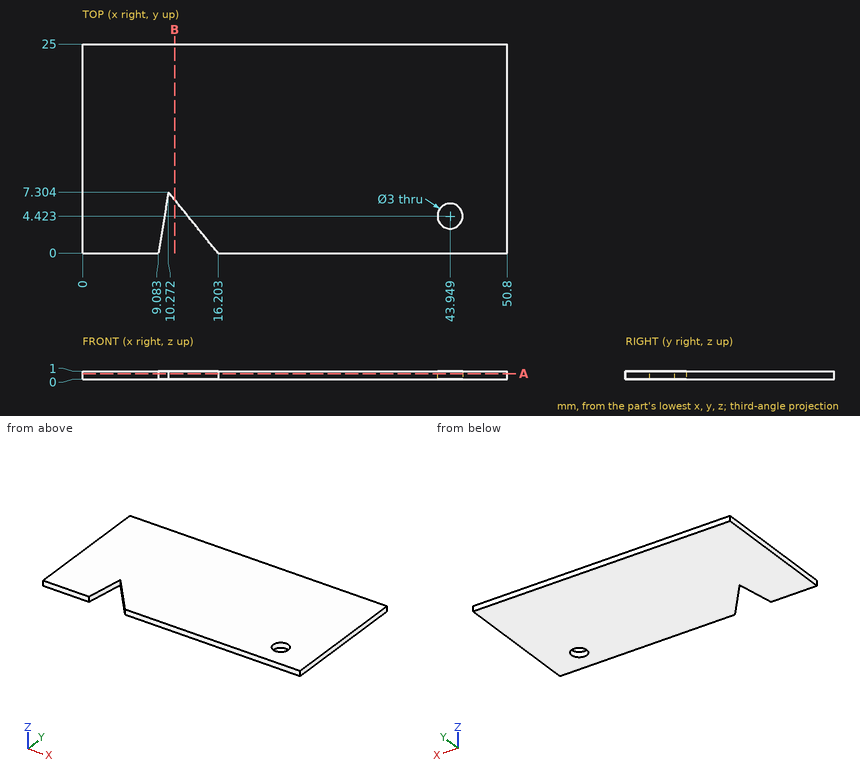
Input: dimensioned drawing with shaded views. Units: mm. Origin: part minimum x, y, z. Coordinates: 2 decimals unless noted, no trailing zeros. Order: outer loops, then holes, each group sorted by start corner. A loop starts at its lowest first (then second) coordinate and runs counter-clockwise, first axis right, second up.
Item 1: Section query B-B (x = 11). Output: boundary loops of the cut face in (y, z), then the cut area to 3 significant figures.
Answer:
outline: (6.41, 0) - (25, 0) - (25, 1) - (6.41, 1) - close
area: 18.6 mm2
Item 2: Section query A-A (z = 0.7). Output: boundary loops of the cut face in (x, y) (1 decimal), then the cut area to 3 significant figures.
Answer:
outline: (0, 0) - (9.1, 0) - (10.3, 7.3) - (16.2, 0) - (50.8, 0) - (50.8, 25) - (0, 25) - close; hole circle Ø3 at (43.9, 4.4)
area: 1,240 mm2
Item 3: Material intervals for line 1 along Y through (x, z) = (45, 0.8) (1 decimal); line 2 along X through (y, z) = (1.5, 0.45) (1 decimal); line 3 along Y through (x, z) = (12, 0.6) (1 decimal), sorted ascending.
Answer:
line 1: y = 0 to 3.4, 5.5 to 25
line 2: x = 0 to 9.3, 15 to 50.8
line 3: y = 5.2 to 25
